Work out the finished part from the listing and answer in its coordinate system (mm). A direction names the side the tool comes from. Give positions to 0.01 mm unless a question says otherwise; leave off trailing zeros. Order: outer loops, then holes, each group sorted by start corner. A loop starts at its lowest first (then second) coordinate and runs counter-clockwise, first axis right, second up. Notation, with made-up numbers: (-35.75, 50.5) -> (-6.75, 50.5) arc R29 ccw to (-6.75, 82.5) -> close; hole circle Ø10 at (80.5, 9.5). An arc over 180 degrees is marked (long way). Answer as CSV lines item,"result". Start each with the question number.
1. A cutting plane is placed at C-C (y = 71.5). Give the vertices of the cut face in (x, z), then the cut area to 3 significant figures.
2. A cutting plane is placed at B-B (z = 87). Give the vertices of the cut face in (x, y).
3. For a pull along Y with two mould halves and no side action, classify faces 4 (the flat face through (96, 38, 5)), 5 (the flat face through (47, -2.5, 47)), 6 (the flat face through (47, 38, 97.5)) as released by +Y, released by -Y, zero draft, split by the parting line, or undercut.
4. For faces 1 (the flat face through (25, 12, 96)), 2 (the flat face through (0, 37, 25)), 3 (the flat face through (22, 0, 7)), determine the directions among +Z, -Z, +X, -X, +Y, -Y from which every point of the face is accessible in a straight line to the end or side of a thin tool.
5. A cutting plane is placed at A-A (y = 38). State how many separate pieces and enclosed holes the cut face has, then the cut area to 3 significant figures.
6. Find the intervals of material crossed by L1, parallel to Y at x = 27, z = 76.5; L2, parallel to X at y = 70.5, z = 57; L3, parallel to Z at x = 84.5, y = 4, in increasing order.
7. A cutting plane is placed at D-D (x = 89.5). Give the vertices of the cut face in (y, z).
from build123d import *

# Parameters (mm, degrees)
BOX006_W           = 9
BOX006_H           = 75
BOX006_DEPTH       = 45
BOX002_W           = 40
BOX002_H           = 50
BOX002_DEPTH       = 5
BOX001_W           = 95
BOX001_H           = 75
BOX001_DEPTH       = 95
BOX_W              = 100
BOX_H              = 80
BOX_DEPTH          = 100
BOX003_W           = 84
BOX003_H           = 75
BOX003_DEPTH       = 4
BOX003_PITCH_ANGLE = -15
BOX004_W           = 3
BOX004_H           = 75
BOX004_DEPTH       = 5
BOX005_W           = 69
BOX005_H           = 75
BOX005_DEPTH       = 4
BOX005_PITCH_ANGLE = 18


with BuildPart() as cube005:
    # Box006 → Box006 (new body)
    with BuildSketch(Plane(origin=(94, 0, 5), x_dir=(1, 0, 0), z_dir=(0, 0, 1))):
        with Locations((4.5, 37.5)):
            Rectangle(BOX006_W, BOX006_H)
    extrude(amount=BOX006_DEPTH)


with BuildPart() as cube001:
    # Box002 → Box002 (new body)
    with BuildSketch(Plane(origin=(5, 12, 94), x_dir=(1, 0, 0), z_dir=(0, 0, 1))):
        with Locations((20, 25)):
            Rectangle(BOX002_W, BOX002_H)
    extrude(amount=BOX002_DEPTH)


with BuildPart() as inside_hole:
    # Box001 → Box001 (new body)
    with BuildSketch(Plane.XY):
        with Locations((47.5, 37.5)):
            Rectangle(BOX001_W, BOX001_H)
    extrude(amount=BOX001_DEPTH)


with BuildPart() as cut001:
    # Box → Box (new body)
    with BuildSketch(Plane(origin=(-2.5, -2.5, -2.5), x_dir=(1, 0, 0), z_dir=(0, 0, 1))):
        with Locations((50, 40)):
            Rectangle(BOX_W, BOX_H)
    extrude(amount=BOX_DEPTH)

    # Cut: cut inside hole
    add(inside_hole.part, mode=Mode.SUBTRACT)

    # Cut001: cut Cube001
    add(cube001.part, mode=Mode.SUBTRACT)


with BuildPart() as fusion:
    # Box003 → Box003 (new body)
    with BuildSketch(Plane.XY):
        with Locations((42, 37.5)):
            Rectangle(BOX003_W, BOX003_H)
    extrude(amount=BOX003_DEPTH)


with BuildPart() as fusion_1:
    # Box003 pitch: moved
    add(fusion.part.rotate(Axis((0, 0, 0), (0, 1, 0)), BOX003_PITCH_ANGLE))


with BuildPart() as fusion_2:
    # Box003 placement: moved
    add(fusion_1.part.moved(Location((15, 0, 29))))

    # Fusion: union Cut001
    add(cut001.part)


with BuildPart() as fusion001:
    # Box004 → Box004 (new body)
    with BuildSketch(Plane.XY.offset(28)):
        with Locations((1.5, 37.5)):
            Rectangle(BOX004_W, BOX004_H)
    extrude(amount=BOX004_DEPTH)

    # Fusion001: union Fusion
    add(fusion_2.part)


with BuildPart() as compartment:
    # Box005 → Box005 (new body)
    with BuildSketch(Plane.XY):
        with Locations((34.5, 37.5)):
            Rectangle(BOX005_W, BOX005_H)
    extrude(amount=BOX005_DEPTH)


with BuildPart() as compartment_1:
    # Box005 pitch: moved
    add(compartment.part.rotate(Axis((0, 0, 0), (0, 1, 0)), BOX005_PITCH_ANGLE))


with BuildPart() as compartment_2:
    # Box005 placement: moved
    add(compartment_1.part.moved(Location((-2, 0, 19))))

    # Fusion002: union Fusion001
    add(fusion001.part)

    # Cut002: cut Cube005
    add(cube005.part, mode=Mode.SUBTRACT)


solid = compartment_2.part
Answer sheet:
1,outline,"(-2.5, -2.5) -> (97.5, -2.5) -> (97.5, 5) -> (95, 5) -> (95, 0) -> (64.38, 0) -> (64.86, 1.48) -> (0, 22.56) -> (0, 28) -> (3, 28) -> (3, 33) -> (0, 33) -> (0, 95) -> (95, 95) -> (95, 54.58) -> (13.96, 32.86) -> (15, 29) -> (95, 50.44) -> (95, 50) -> (97.5, 50) -> (97.5, 97.5) -> (-2.5, 97.5) -> close; hole (0, 0) -> (56.48, 0) -> (0, 18.35) -> close"
1,area,"1,470 mm^2"
2,outline,"(-2.5, -2.5) -> (97.5, -2.5) -> (97.5, 77.5) -> (-2.5, 77.5) -> close; hole (0, 0) -> (95, 0) -> (95, 75) -> (0, 75) -> close"
3,face 4,"undercut"
3,face 5,"released by -Y"
3,face 6,"zero draft"
4,face 1,"+Z"
4,face 2,"+X"
4,face 3,"none"
5,separate pieces,"2"
5,enclosed holes,"1"
5,area,"1,370 mm^2"
6,L1,"y = -2.5 to 0, 75 to 77.5"
6,L2,"x = -2.5 to 0, 95 to 97.5"
6,L3,"z = -2.5 to 0, 47.62 to 51.76, 95 to 97.5"
7,outline,"(-2.5, -2.5) -> (77.5, -2.5) -> (77.5, 97.5) -> (-2.5, 97.5) -> close; hole (0, 0) -> (75, 0) -> (75, 48.96) -> (0, 48.96) -> close; hole (0, 53.1) -> (75, 53.1) -> (75, 95) -> (0, 95) -> close"
